```python
from build123d import *

# Parameters (mm, degrees)
EXTRUDE_1_DEPTH     = 3
SKETCH_2_W          = 60
SKETCH_2_H          = 30
CUT_EXTRUDE_2_DEPTH = 417.901436616
SKETCH_3_R          = 16
SKETCH_3_R_2        = 2.25
SKETCH_3_R_3        = 5
CUT_EXTRUDE_3_DEPTH = 417.901436616
EXTRUDE_START       = -3
EXTRUDE_4_DEPTH     = 3


with BuildPart() as part:
    # 草圖1 → 伸長1 (new body)
    with BuildSketch(Plane.XY):
        with BuildLine():
            Line((55.280581326, 100), (374.719418674, 100))
            ThreePointArc((374.719418674, 100), (401.086913014, 84.309271198), (399.872727163, 53.650349482))
            Line((399.872727163, 53.650349482), (373.872727163, 13.650349482))
            ThreePointArc((373.872727163, 13.650349482), (363.028689873, 3.63250566), (348.719418674, 0))
            Line((348.719418674, 0), (81.280581326, 0))
            ThreePointArc((81.280581326, 0), (66.971310127, 3.63250566), (56.127272837, 13.650349482))
            Line((56.127272837, 13.650349482), (30.127272837, 53.650349482))
            ThreePointArc((30.127272837, 53.650349482), (28.913086986, 84.309271198), (55.280581326, 100))
        make_face()
    extrude(amount=EXTRUDE_1_DEPTH)

    # 草圖2 → 伸長2 (cut, through all)
    with BuildSketch(Plane.XY.offset(3)):
        with Locations((110, 35)):
            Rectangle(SKETCH_2_W, SKETCH_2_H)
        with Locations((180, 35)):
            Rectangle(SKETCH_2_W, SKETCH_2_H)
        with Locations((250, 35)):
            Rectangle(SKETCH_2_W, SKETCH_2_H)
        with Locations((320, 35)):
            Rectangle(SKETCH_2_W, SKETCH_2_H)
    extrude(amount=-CUT_EXTRUDE_2_DEPTH, mode=Mode.SUBTRACT)

    # 草圖3 → 伸長3 (cut, through all)
    with BuildSketch(Plane.XY.offset(3)):
        with Locations((55.280581326, 70)):
            Circle(SKETCH_3_R)
        with Locations((55.280581326, 90)):
            Circle(SKETCH_3_R_2)
        with Locations((75.280581326, 70)):
            Circle(SKETCH_3_R_2)
        with Locations((55.280581326, 50)):
            Circle(SKETCH_3_R_2)
        with Locations((35.280581326, 70)):
            Circle(SKETCH_3_R_2)
        with Locations((374.719418674, 70)):
            Circle(SKETCH_3_R_3)
    extrude(amount=-CUT_EXTRUDE_3_DEPTH, mode=Mode.SUBTRACT)

    # 草圖4 → 伸長4 (add)
    with BuildSketch(Plane.XY.offset(3).offset(EXTRUDE_START)):
        with BuildLine():
            Line((399.872727163, 53.650349482), (391, 40))
            Line((391, 40), (415, 40))
            Line((415, 40), (415, 120))
            Line((415, 120), (15, 120))
            Line((15, 120), (15, 40))
            Line((15, 40), (39, 40))
            Line((39, 40), (30.127272837, 53.650349482))
            ThreePointArc((30.127272837, 53.650349482), (28.913086986, 84.309271198), (55.280581326, 100))
            Line((55.280581326, 100), (374.719418674, 100))
            ThreePointArc((374.719418674, 100), (401.086913014, 84.309271198), (399.872727163, 53.650349482))
        make_face()
    extrude(amount=EXTRUDE_4_DEPTH)


solid = part.part
```
Here's how the part is built. I have some questions about the finished solid (model axes, mm). Coordinates: 2 decimals unless noted, no trailing zeros. Order: outer loops, then holes, each group sorted by start corner. A loop starts at its lowest first (then second) coordinate and runs counter-clockwise, first axis right, second up.
Item 1: If we section it at B-B, the plane z = 2.3: Give the number of separate pieces and of enclosed holes in the cut face, then the cut area to 3 significant figures.
Response values:
separate pieces: 1
enclosed holes: 10
area: 36,800 mm2
Item 2: I'm going to push flat-ended pins straight in: pin 1 Ø1.5 at (y, z) = (35, 1) entering from +X; pin 2 Ø1.5 at (y, z) = (39.5, 1) entering from -X. Where does each tip first touch, or does it pass through?
Response values:
pin 1: stops at x = 388.24
pin 2: stops at x = 15
Item 3: If we section it at A-A, the plane x = 199: List the corners of the cut face in (y, z) for me.
Response values:
outline: (0, 0) - (20, 0) - (20, 3) - (0, 3) - close; (50, 0) - (120, 0) - (120, 3) - (50, 3) - close
Item 4: I need wall thicknesses on probe 1 along X at (y, z) = (69.5, 0.6); probe 2 along Y at (x, z) = (278.5, 0.35); probe 3 along X at (y, z) = (39, 1.85). Which ranges of each line are inside material? Lowest first, please.
Response values:
probe 1: x = 15 to 33.09, 37.47 to 39.29, 71.27 to 73.09, 77.47 to 369.74, 379.69 to 415
probe 2: y = 0 to 20, 50 to 120
probe 3: x = 39.65 to 80, 140 to 150, 210 to 220, 280 to 290, 350 to 390.35
